Read the model definition and answer for the solid it produces. Units are mm, in the model's axes. Round coordinates to 2 decimals unless told otherwise and drop trailing zeros. Write each loop counter-clockwise with the first axis right and the second up, starting at its lowest first coordinate (ties: lowest second). Pieces come first, ordered by that corner, then holes. Notation, with made-up numbers: (55, 12.5) -> (97, 12.5) arc R21 ccw to (97, 21.5) -> close; hole circle Ø4 at (20, -24). An arc over 180 degrees is marked (long way). Return JSON: item names as keys, results as strings. Group by question number.
(1) Given pin 1 (12 mm diameter, centred on x = -41.5, y = -10, fed in from -Z), flat-ended and moving along its own axis, determine where the tip first touches the part or whether it passes through.
(2) A cutting plane is placed at B-B on y = 1. Give the vertices of the cut face in (x, z), then the cut area to 3 significant figures.
(3) A cutting plane is placed at D-D on x = 38.5. Give the vertices of the cut face in (y, z), then the cut area to 3 significant figures.
(4) Straight lines are drawn through the part: line 1 (X direction, y = 38, z = 1.05); line 2 (Y direction, x = -28.5, z = 0.4) (1 decimal); line 3 (Y direction, x = 7, z = 1.4). For each, find the intervals that lie inside material, in ascending order.
(5) A cutting plane is placed at A-A on x = 0. Give the vertices of the cut face in (y, z), then the cut area to 3 significant figures.
(6) A cutting plane is placed at C-C on z = 0.9. Give the vertices of the cut face in (x, y), then the cut area to 3 significant figures.
```python
from build123d import *

# Parameters (mm, degrees)
F1_DEPTH = 2


with BuildPart() as f1:
    # F0 (on Top) → F1 (new body)
    with BuildSketch(Plane.XY):
        with BuildLine():
            ThreePointArc((53, 137), (0, 190), (-53, 137))
            Line((-53, 137), (-53, -137))
            ThreePointArc((-53, -137), (0, -190), (53, -137))
            Line((53, -137), (53, 137))
        make_face()
        with BuildLine():
            Line((-34, -137), (-34, 137))
            ThreePointArc((-34, 137), (0, 171), (34, 137))
            Line((34, 137), (34, -137))
            ThreePointArc((34, -137), (0, -171), (-34, -137))
        make_face(mode=Mode.SUBTRACT)
    extrude(amount=F1_DEPTH)


solid = f1.part
```
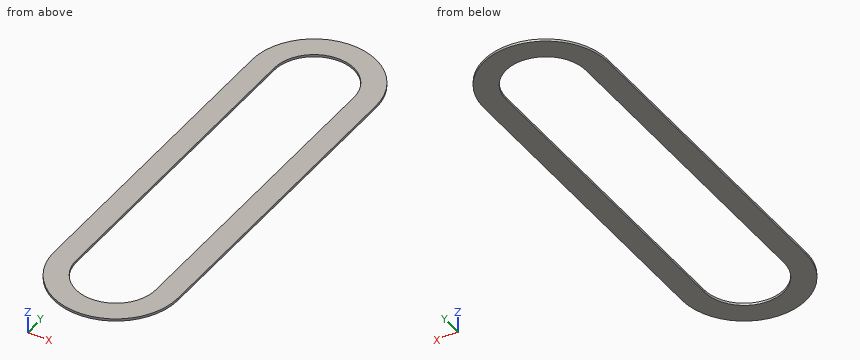
Checks:
{
 "1": {"pin 1": "stops at z = 0"},
 "2": {"outline": "(-53, 0) -> (-34, 0) -> (-34, 2) -> (-53, 2) -> close; (34, 0) -> (53, 0) -> (53, 2) -> (34, 2) -> close", "area": "76.0 mm^2"},
 "3": {"outline": "(-173.42, 0) -> (173.42, 0) -> (173.42, 2) -> (-173.42, 2) -> close", "area": "694 mm^2"},
 "4": {"line 1": "x = -53 to -34, 34 to 53", "line 2": "y = -181.7 to -155.5, 155.5 to 181.7", "line 3": "y = -189.54 to -170.27, 170.27 to 189.54"},
 "5": {"outline": "(-190, 0) -> (-171, 0) -> (-171, 2) -> (-190, 2) -> close; (171, 0) -> (190, 0) -> (190, 2) -> (171, 2) -> close", "area": "76.0 mm^2"},
 "6": {"outline": "(-53, -137) arc R53 ccw to (53, -137) -> (53, 137) arc R53 ccw to (-53, 137) -> close; hole (-34, -137) arc R34 ccw to (34, -137) -> (34, 137) arc R34 ccw to (-34, 137) -> close", "area": "15,600 mm^2"}
}
